Geometry: see drawing. Coordinates: mm, zero at the bounding-box minimum. Coordinates: 2 decimals unless noted, no trailing zeros. Write each loop counter-clockwise with the first axis right and the second up, starting at its lowest first coordinate (ties: lowest second). Pieces come first, ordered by that corner, then holes.
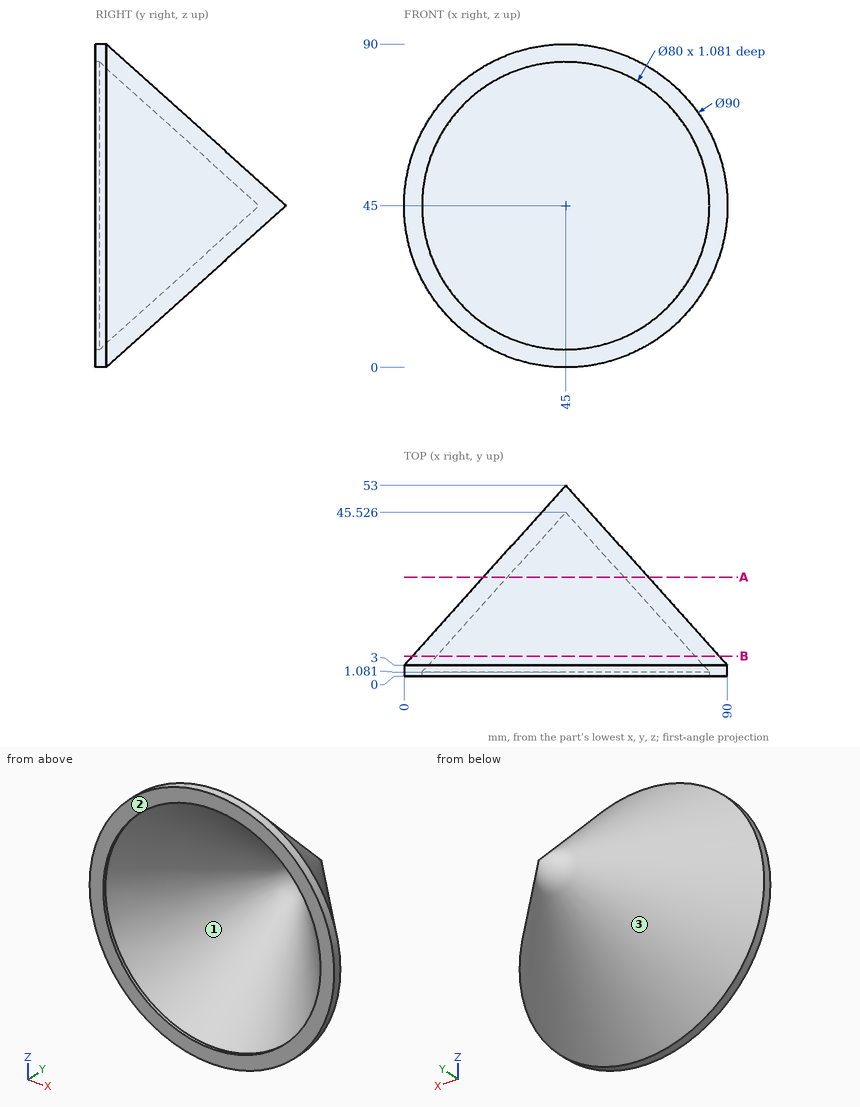
Item 1: Pull-direction query (X, two-part tool) for the marked faces 1, 2 and 3; classes: released by +X, released by -X, zero draft, split by the parting line, or undercut.
Derived:
face 1: undercut
face 2: zero draft
face 3: split by the parting line
Item 2: Section B-B, the plane y = 5.5. Output: boundary loops of the cut face in (x, z).
Derived:
outline: circle Ø85.5 at (45, 45); hole circle Ø72.05 at (45, 45)
Item 3: Section A-A, the plane y = 27.5. Output: boundary loops of the cut face in (x, z).
Derived:
outline: circle Ø45.9 at (45, 45); hole circle Ø32.45 at (45, 45)
Item 4: Material intervals for probe 1 along Z at (x, y) = (45, 0.55); probe 2 along Z at (x, y) = (54, 11.5); probe 3 along X at (y, z) = (37, 51) (1 decimal), sorted ascending.
Derived:
probe 1: z = 0 to 5, 85 to 90
probe 2: z = 8.75 to 15.73, 74.27 to 81.25
probe 3: x = 31.9 to 40.2, 49.8 to 58.1
Item 5: Pin query (flat end, axial travel): pin 1 (8 mm diameter, centred on y = 17, z = 54.5, fed in from -X) (1 decimal); pin 2 (5 mm diameter, centred on x = 35.5, y = 9, fed in from +Z) (1 decimal); pin 3 (2 mm diameter, centred on y = 22, z = 43.5, fed in from +X). Return the tip coordinate at first contact, or that it passes through.
Derived:
pin 1: stops at x = 10.1
pin 2: stops at z = 85.8
pin 3: stops at x = 73.76
